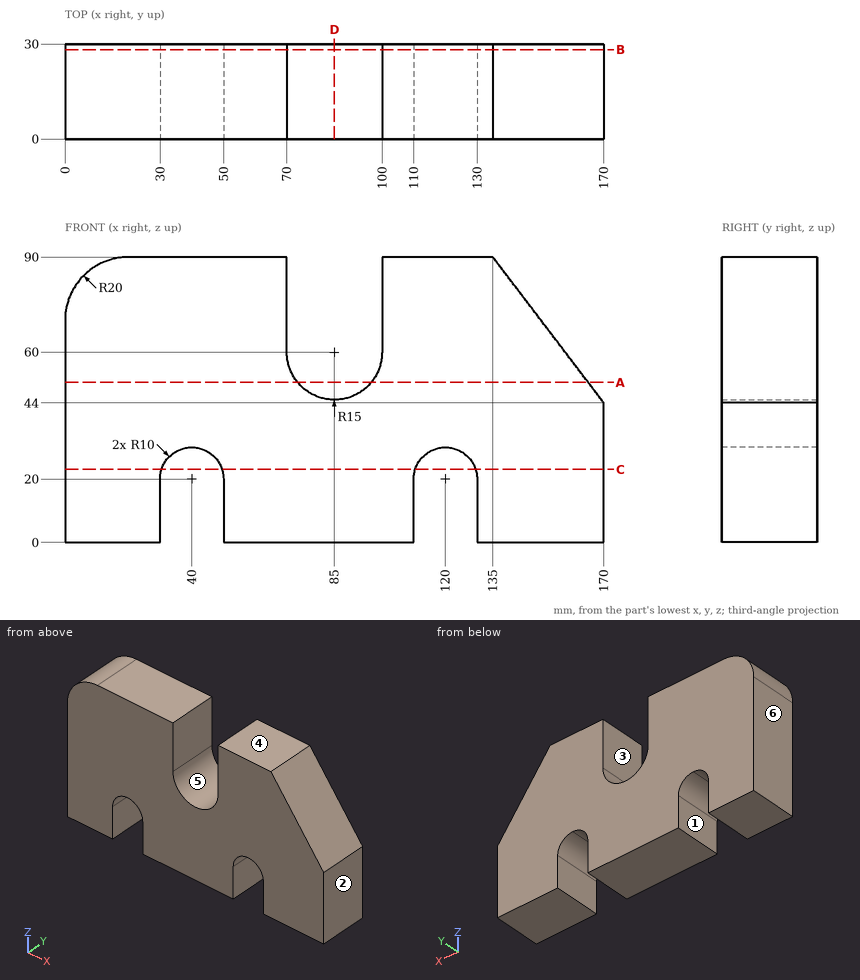
Geometry: see drawing. Coordinates: mm, zero at the bounding-box minimum. A direction names the side the tool comes from. Give positions to 0.01 mm unless a question says otherwise; leave off trailing zeros. Order: outer loops, then holes, each group sorted by start corner. A loop starts at its lowest first (then second) coordinate and runs counter-clockwise, first axis right, second up. Notation, with made-up numbers: (43.5, 24) - (48.5, 24) arc R19 ccw to (48.5, 29) - close; hole circle Ø7 at (19, -35). An arc over 180 degrees is marked (long way). One line per item, written item: value.
1. Cut plane A-A, the plane z = 50.5. Output: boundary loops of the cut face in (x, y).
Determined:
outline: (0, 0) - (73.39, 0) - (73.39, 30) - (0, 30) - close; (96.61, 0) - (165.05, 0) - (165.05, 30) - (96.61, 30) - close
2. Cut plane B-B, the plane y = 28.25. Output: boundary loops of the cut face in (x, z).
Determined:
outline: (0, 0) - (30, 0) - (30, 20) arc R10 cw to (40, 30) arc R10 cw to (50, 20) - (50, 0) - (110, 0) - (110, 20) arc R10 cw to (120, 30) arc R10 cw to (130, 20) - (130, 0) - (170, 0) - (170, 44) - (135, 90) - (100, 90) - (100, 60) arc R15 cw to (70, 60) - (70, 90) - (20, 90) arc R20 ccw to (0, 70) - close
3. Pin query (flat end, axial travel): pin 1 Ø5 at (y, z) = (21, 49.5) entering from +X; pin 2 Ø9 at (y, z) = (10, 78.5) entering from +X. Return the tip coordinate at first contact, or that it passes through.
Determined:
pin 1: x = 167.72
pin 2: x = 147.17
4. Reachability of the marked faces 1, 2 and 3 from +Z, -Z, +X, -X, +Y, -Y: full face, straight path, thin tool, end or side. Return the list, or none.
Determined:
face 1: -Z, +Y, -Y
face 2: +Z, -Z, +X, +Y, -Y
face 3: +Z, +Y, -Y
5. Line query: probe 1 along X at (y, z) = (26.25, 5.5); probe 2 along X at (y, z) = (12.25, 68); probe 3 along Z at (x, y) = (84, 9.5). Output: solid intervals per line, ascending.
Determined:
probe 1: 0 to 30, 50 to 110, 130 to 170
probe 2: 0 to 70, 100 to 151.74
probe 3: 0 to 45.03
6. Cut plane C-C, the plane z = 23. Output: boundary loops of the cut face in (x, y), and give its area (3 significant figures).
Determined:
outline: (0, 0) - (30.46, 0) - (30.46, 30) - (0, 30) - close; (49.54, 0) - (110.46, 0) - (110.46, 30) - (49.54, 30) - close; (129.54, 0) - (170, 0) - (170, 30) - (129.54, 30) - close
area: 3,960 mm2
7. Cut plane D-D, the plane x = 85. Output: boundary loops of the cut face in (y, z), and give its area (3 significant figures).
Determined:
outline: (0, 0) - (30, 0) - (30, 45) - (0, 45) - close
area: 1,350 mm2
8. Draft query along X for the marked faces 4, 5 and 6. Return one class per face: released by +X, released by -X, zero draft, split by the parting line, or undercut.
Determined:
face 4: zero draft
face 5: undercut
face 6: released by -X
